from build123d import *

# Parameters (mm, degrees)
SKETCH2_W            = 26
SKETCH2_H            = 23.3
BOSS_EXTRUDE1_DEPTH  = 20
SKETCH3_W            = 14.5
SKETCH3_H            = 5.7
CUT_EXTRUDE1_DEPTH   = 20
SKETCH4_W            = 10.09
SKETCH4_H            = 4.9
CUT_EXTRUDE2_DEPTH   = 17.5
SKETCH5_W            = 10.09
SKETCH5_H            = 4.9
CUT_EXTRUDE3_DEPTH   = 17.5
SKETCH10_W           = 3
SKETCH10_H           = 2
CUT_EXTRUDE4_DEPTH   = 17.5
SKETCH11_W           = 3
SKETCH11_H           = 2
CUT_EXTRUDE5_DEPTH   = 17.5
SKETCH7_W            = 19
SKETCH7_H            = 1.78
CUT_EXTRUDE6_DEPTH   = 18.5
SKETCH6_W            = 19
SKETCH6_H            = 1.78
CUT_EXTRUDE7_DEPTH   = 18.5
SKETCH9_W            = 15.8
SKETCH9_H            = 2.12
CUT_EXTRUDE8_DEPTH   = 17.5
SKETCH12_W           = 15.8
SKETCH12_H           = 2.12
CUT_EXTRUDE9_DEPTH   = 17.5
SKETCH14_W           = 7.8
SKETCH14_H           = 20
BOSS_EXTRUDE2_DEPTH  = 6
SKETCH13_W           = 20
SKETCH13_H           = 12
BOSS_EXTRUDE3_DEPTH  = 20
SKETCH15_R           = 3.05
CUT_EXTRUDE10_DEPTH  = 19
SKETCH16_W           = 4
SKETCH16_H           = 15
CUT_EXTRUDE11_DEPTH  = 20
SKETCH18_W           = 4
SKETCH18_H           = 9
CUT_EXTRUDE12_DEPTH  = 20
BOSS_EXTRUDE8_DEPTH  = 32.5
BOSS_EXTRUDE9_DEPTH  = 32.5
SKETCH23_W           = 10
SKETCH23_H           = 20
CUT_EXTRUDE14_DEPTH  = 6
SKETCH24_W           = 24
SKETCH24_H           = 20
BOSS_EXTRUDE10_DEPTH = 1.4
SKETCH26_R           = 1.45
CUT_EXTRUDE15_DEPTH  = 10


with BuildPart() as part:
    # Sketch2 → Boss-Extrude1 (new body)
    with BuildSketch(Plane.XY):
        Rectangle(SKETCH2_W, SKETCH2_H)
    extrude(amount=BOSS_EXTRUDE1_DEPTH)

    # Sketch3 → Cut-Extrude1 (cut)
    with BuildSketch(Plane.XY.offset(20)):
        Rectangle(SKETCH3_W, SKETCH3_H)
    extrude(amount=-CUT_EXTRUDE1_DEPTH, mode=Mode.SUBTRACT)

    # Sketch4 → Cut-Extrude2 (cut)
    with BuildSketch(Plane.XY.offset(20)):
        with Locations((0, 5.3)):
            Rectangle(SKETCH4_W, SKETCH4_H)
    extrude(amount=-CUT_EXTRUDE2_DEPTH, mode=Mode.SUBTRACT)

    # Sketch5 → Cut-Extrude3 (cut)
    with BuildSketch(Plane.XY.offset(20)):
        with Locations((0, -5.3)):
            Rectangle(SKETCH5_W, SKETCH5_H)
    extrude(amount=-CUT_EXTRUDE3_DEPTH, mode=Mode.SUBTRACT)

    # Sketch10 → Cut-Extrude4 (cut)
    with BuildSketch(Plane.XY.offset(20)):
        with Locations((9.1, 6.75)):
            Rectangle(SKETCH10_W, SKETCH10_H)
    extrude(amount=-CUT_EXTRUDE4_DEPTH, mode=Mode.SUBTRACT)

    # Sketch11 → Cut-Extrude5 (cut)
    with BuildSketch(Plane.XY.offset(20)):
        with Locations((-9.1, -6.75)):
            Rectangle(SKETCH11_W, SKETCH11_H)
    extrude(amount=-CUT_EXTRUDE5_DEPTH, mode=Mode.SUBTRACT)

    # Sketch7 → Cut-Extrude6 (cut)
    with BuildSketch(Plane.XY.offset(20)):
        with Locations((-2.3, -8.64)):
            Rectangle(SKETCH7_W, SKETCH7_H)
    extrude(amount=-CUT_EXTRUDE6_DEPTH, mode=Mode.SUBTRACT)

    # Sketch6 → Cut-Extrude7 (cut)
    with BuildSketch(Plane.XY.offset(20)):
        with Locations((2.3, 8.64)):
            Rectangle(SKETCH6_W, SKETCH6_H)
    extrude(amount=-CUT_EXTRUDE7_DEPTH, mode=Mode.SUBTRACT)

    # Sketch9 → Cut-Extrude8 (cut)
    with BuildSketch(Plane.XY.offset(20)):
        with Locations((2.7, 10.59)):
            Rectangle(SKETCH9_W, SKETCH9_H)
    extrude(amount=-CUT_EXTRUDE8_DEPTH, mode=Mode.SUBTRACT)

    # Sketch12 → Cut-Extrude9 (cut)
    with BuildSketch(Plane.XY.offset(20)):
        with Locations((-2.7, -10.59)):
            Rectangle(SKETCH12_W, SKETCH12_H)
    extrude(amount=-CUT_EXTRUDE9_DEPTH, mode=Mode.SUBTRACT)

    # Sketch14 → Boss-Extrude2 (add)
    with BuildSketch(Plane(origin=(0, 11.65, 0), x_dir=(1, 0, 0), z_dir=(0, 1, 0))):
        with Locations((-9.1, -10)):
            Rectangle(SKETCH14_W, SKETCH14_H)
    extrude(amount=BOSS_EXTRUDE2_DEPTH)

    # Sketch13 → Boss-Extrude3 (add)
    with BuildSketch(Plane.ZY.offset(13)):
        with Locations((10, 11.65)):
            Rectangle(SKETCH13_W, SKETCH13_H)
    extrude(amount=BOSS_EXTRUDE3_DEPTH)

    # Sketch15 → Cut-Extrude10 (cut)
    with BuildSketch(Plane.XY.offset(20)):
        with Locations((-26.1, 11.65)):
            Circle(SKETCH15_R)
    extrude(amount=-CUT_EXTRUDE10_DEPTH, mode=Mode.SUBTRACT)

    # Sketch16 → Cut-Extrude11 (cut)
    with BuildSketch(Plane.XY.offset(20)):
        with Locations((11, -4.15)):
            Rectangle(SKETCH16_W, SKETCH16_H)
    extrude(amount=-CUT_EXTRUDE11_DEPTH, mode=Mode.SUBTRACT)

    # Sketch18 → Cut-Extrude12 (cut)
    with BuildSketch(Plane.XY.offset(20)):
        with Locations((-11, 1.15)):
            Rectangle(SKETCH18_W, SKETCH18_H)
    extrude(amount=-CUT_EXTRUDE12_DEPTH, mode=Mode.SUBTRACT)

    # Sketch21 → Boss-Extrude8 (add)
    with BuildSketch(Plane.XY.offset(20)):
        Polygon((-13, -11.65), (-13, -3.35), (-10.6, -3.35), (-10.6, -7.75), (-11.8, -7.75), (-11.8, -9.53), (-10.6, -9.53), (-10.6, -11.65), align=None)
        Polygon((5.2, -9.53), (5.2, -11.65), (9, -11.65), (9, -4.25), (5.045, -4.25), (5.045, -7.75), (7.2, -7.75), (7.2, -9.53), align=None)
    extrude(amount=BOSS_EXTRUDE8_DEPTH)

    # Sketch22 → Boss-Extrude9 (add)
    with BuildSketch(Plane.XY.offset(20)):
        Polygon((10.6, 11.65), (13, 11.65), (13, 3.35), (10.6, 3.35), (10.6, 7.75), (11.8, 7.75), (11.8, 9.53), (10.6, 9.53), align=None)
        Polygon((-5.2, 9.53), (-5.2, 11.65), (-9, 11.65), (-9, 4.25), (-5.045, 4.25), (-5.045, 7.75), (-7.2, 7.75), (-7.2, 9.53), align=None)
    extrude(amount=BOSS_EXTRUDE9_DEPTH)

    # Sketch23 → Cut-Extrude14 (cut)
    with BuildSketch(Plane(origin=(0, 17.65, 0), x_dir=(1, 0, 0), z_dir=(0, 1, 0))):
        with Locations((-10.2, -10)):
            Rectangle(SKETCH23_W, SKETCH23_H)
    extrude(amount=-CUT_EXTRUDE14_DEPTH, mode=Mode.SUBTRACT)

    # Sketch24 → Boss-Extrude10 (add)
    with BuildSketch(Plane.XZ.offset(-5.65)):
        with Locations((-21, 10)):
            Rectangle(SKETCH24_W, SKETCH24_H)
    extrude(amount=BOSS_EXTRUDE10_DEPTH)

    # Sketch26 → Cut-Extrude15 (cut)
    with BuildSketch(Plane(origin=(0, 0, 0), x_dir=(-1, 0, 0), z_dir=(0, 0, -1))):
        with Locations((26.1, 11.65)):
            Circle(SKETCH26_R)
    extrude(amount=-CUT_EXTRUDE15_DEPTH, mode=Mode.SUBTRACT)


solid = part.part
Geometry: final body of the model. Coordinates: model frame, mm. A direction names the side the tool comes from. Give positions to 0.01 mm unless a question says otherwise; leave off trailing zeros. Loops run counter-clockwise (first coordinate to the right, second up) from the corner with the lowest first, then second, coordinate; pieces in that order, holes last. Notation, with made-up numbers: M 24.25,-5.75 L 32.25,-5.75 A26 ccw 32.25,13.25 Z; hole C 76.5,-35 d2. An arc over 180 degrees is marked long. Put each result on its own line as item: value. Start each with the question number.
1) Ray query, line 1 along Y through (x, z) = (-26, 12); line 2 along X through (y, z) = (-7.5, 17) (3 decimals); line 3 along X through (y, z) = (-8.5, 3.5). Return the intervals inside material, ascending.
2) Access query for faces 4 (the flat face through (-3, -11, 2.5)), 5 (the flat face through (10.6, 11, 27)), 6 (the flat face through (0, 5, 2.5)). Directions: +Z, -Z, +X, -X, +Y, -Y. A direction counts if a zero-diameter tool reaches every point of the face in a straight line with its end or side. Return the directions, or none.
3) Cut plane B-B (x = -26.1). Output: boundary loops of the cut face in (y, z).
4) Contact query for flat-ended pins moving along their axis: pin 1 (4 mm diameter, centred on x = -3, y = 8, fed in from +Z); pin 2 (8 mm diameter, centred on x = -20, y = 7, fed in from +Z); pin 3 (6 mm diameter, centred on y = 10, z = 30, fed in from -X); pin 4 (4 mm diameter, centred on y = -1, z = 41.5, fed in from -X). Output: stop coordinate, or through.
5) Pull-direction query (X, two-part tool) for faces 1 (the flat face through (-9, 0, 10)), 2 (the flat face through (3, 11, 2.5)), 3 (the flat face through (7.4, -7.9, 52.5)); classes: pulls with the +X half, pulls with the -X half, needs draft (parallel to the pull), parting line crosses it, or undercut.
6) Cut plane C-C (y = -0.5). Output: boundary loops of the cut face in (x, z), then the cut area to 3 significant figures.
7) Cut plane A-A (z = 27.5). Give the number of separate pieces and of enclosed holes in the cut face, then the cut area to 3 significant figures.
Verdict:
1. line 1: 4.25 to 8.6, 14.7 to 17.65
1. line 2: -13 to -10.6, -7.6 to -5.045, 5.045 to 9
1. line 3: -13 to -11.8, 7.2 to 9
2. face 4: +Z, -Y
2. face 5: +Z, +Y
2. face 6: +Z, +Y, -Y
3. outline: M 4.25,0 L 10.2,0 L 10.2,1 L 8.6,1 L 8.6,20 L 4.25,20 Z; M 13.1,0 L 17.65,0 L 17.65,20 L 14.7,20 L 14.7,1 L 13.1,1 Z
4. pin 1: z = 2.5
4. pin 2: z = 20
4. pin 3: x = -9
4. pin 4: through
5. face 1: pulls with the -X half
5. face 2: undercut
5. face 3: needs draft
6. outline: M -9,0 L -7.25,0 L -7.25,20 L -9,20 Z; M 7.25,0 L 9,0 L 9,20 L 7.25,20 Z
6. area: 70.0 mm2
7. separate pieces: 4
7. enclosed holes: 0
7. area: 85.8 mm2
